```python
from build123d import *

# Parameters (mm, degrees)
F0_R     = 52.884546
F0_R_2   = 33.012326
F1_DEPTH = 25
F2_W     = 7.556897
F2_H     = 29.523836
F3_DEPTH = 25
F4_R     = 11.814692
F5_DEPTH = 25


with BuildPart() as f1:
    # F0 (on Top) → F1 (new body)
    with BuildSketch(Plane.XY):
        with Locations((-60.435541, 15.276187)):
            Circle(F0_R)
        with Locations((-55.982087, 15.276187)):
            Circle(F0_R_2, mode=Mode.SUBTRACT)
    extrude(amount=F1_DEPTH)

    # F2 (on face) → F3 (cut)
    with BuildSketch(Plane(origin=(0, 0, 0), x_dir=(1, 0, 0), z_dir=(0, 0, -1))):
        with Locations((-91.813431, -22.13712)):
            Rectangle(F2_W, F2_H)
    extrude(amount=-F3_DEPTH, mode=Mode.SUBTRACT)

    # F4 (on face) → F5 (cut)
    with BuildSketch(Plane(origin=(0, 0, 0), x_dir=(1, 0, 0), z_dir=(0, 0, -1))):
        with Locations((-88.034983, -7.375202)):
            Circle(F4_R)
    extrude(amount=-F5_DEPTH, mode=Mode.SUBTRACT)


solid = f1.part
```
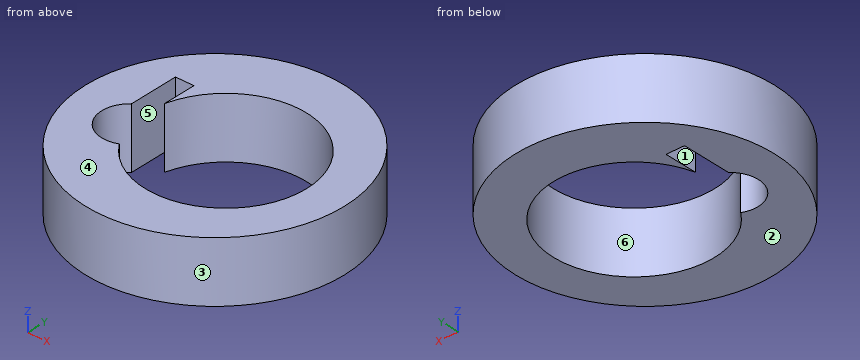
Could you check a few things on this model? Use its own coordinates, in mm. Face numbers are marked on the shaded views. A direction names the side the tool comes from. Give positions to 0.01 mm unless a question says otherwise; leave off trailing zeros. Order: outer loops, then holes, each group sorted by start corner. A loop starts at its lowest first (then second) coordinate and runs counter-clockwise, first axis right, second up.
Q1. I'm going to push flat-ended pins straight in: P1, Ø1.5, axis at x = -27, z = 14, coming from the -Y side; P2, Ø2.5, axis at x = -92.5, z = 7, coming from the -Y side; P3, Ø3, axis at x = -59, z = 17, coming from the -Y side. Where does each tip first touch, or does it pass through?
Q2. Suppose I cut it at A-A, the plane x = -44. Write out the boundary of the cut face in (y, z), and give its area (3 significant figures).
Q3. If I drill on line 1 along X through (y, z) = (16.5, 10.5); line 2 along X through (y, z) = (28, 13.25); line 3 along Y through (x, z) = (-84.5, 12), over which ranges is the centre line in solid material (lowest first)?
Q4. We'd pull the mould along Y, two halves only. Please class the marked faces 3, 4, 5 and 6: +Y half, -Y half, draft (parallel to the pull), parting line (faces both ways), or undercut.
Q5. For the marked faces 1 and 2, which set-ups out of +Z, -Z, +X, -X, +Y, -Y let a thin tool reach every point of the face, with its end or its side?
Q6. Suppose I cut it at B-B, the plane y = 25.5. Write out the boundary of the cut face in (x, z).
Q7. Suppose I cut it at C-C, the plane y = 39. Write out the boundary of the cut face in (x, z), and give its area (3 significant figures).
Q8. Suppose I cut it at D-D, the plane z = 7. Write out the boundary of the cut face in (x, y).
Solution:
1. P1: stops at y = -26.3
1. P2: stops at y = -27.7
1. P3: stops at y = -37.61
2. outline: (-34.99, 0) - (-15.48, 0) - (-15.48, 25) - (-34.99, 25) - close; (46.04, 0) - (65.54, 0) - (65.54, 25) - (46.04, 25) - close
2. area: 975 mm2
3. line 1: x = -113.31 to -95.59, -22.99 to -7.57
3. line 2: x = -111.77 to -95.59, -88.03 to -86.44, -25.52 to -9.1
3. line 3: y = -31.82 to -3.9, 31.91 to 62.37
4. face 3: parting line
4. face 4: draft
4. face 5: undercut
4. face 6: undercut
5. face 1: +Z, -Z
5. face 2: -Z, +X, -X, +Y, -Y
6. outline: (-112.32, 0) - (-95.59, 0) - (-95.59, 25) - (-112.32, 25) - close; (-88.03, 0) - (-87.37, 0) - (-87.37, 25) - (-88.03, 25) - close; (-24.59, 0) - (-8.55, 0) - (-8.55, 25) - (-24.59, 25) - close
7. outline: (-107.7, 0) - (-78.94, 0) - (-78.94, 25) - (-107.7, 25) - close; (-33.03, 0) - (-13.17, 0) - (-13.17, 25) - (-33.03, 25) - close
7. area: 1,220 mm2
8. outline: circle Ø105.77 at (-60.44, 15.28); hole (-95.59, 16.46) arc R11.81 ccw to (-83.2, -3.4) arc R33.01 ccw (long way) to (-88.03, 23.18) - (-88.03, 36.9) - (-95.59, 36.9) - close
